Read the model definition and answer for the solid it produces. Units are mm, in the model's axes. A direction names the side the tool comes from. Coordinates: 2 decimals unless noted, no trailing zeros. Order: outer loops, then holes, each group sorted by start corner. A loop starts at its lowest first (then second) coordinate and runs counter-clockwise, first axis right, second up. Notation, with made-up numbers: (80, 12.5) -> (121, 12.5) arc R31 ccw to (121, 38.5) -> close; hole circle Ø6 at (72.25, 3.25). An arc over 180 degrees is marked (long way). Answer as a JSON object with one key per item and string values. Group by question number.
1) Determine the mould class of faces 3 (the flat face through (1.029, -5, 16)), 4 (the flat face through (-1, -1, 31.75)), 5 (the cylindrical face through (1.31, -7, 29.88)) for opening direction Z: released by +Z, released by -Z, zero draft, split by the parting line, or undercut.
2) Section C-C on y = -4.75 is taken. Determine the outline of the cut face in (x, z).
3) Consider L1, parallel to Z at x = 0, y = 1; L2, parallel to Y at x = -5.75, z = 17. Determine where each line is inside the solid, lowest interval first.
4) Given pin 1 (6.5 mm diameter, centred on x = -6, z = 16.5, fed in from -Y); pin 2 (2.5 mm diameter, centred on x = 0, y = -2, fed in from -Z); pin 3 (4 mm diameter, centred on y = -6, z = 13.5, fed in from -X), each flat-ended and moving along its own axis, determine where each tip first touches the part or whether it passes through.
5) Section D-D on z = 8.5 is taken. Determine the outline of the cut face in (x, y) (1 decimal).
6) Section A-A on z = 13.5 is taken. Determine the outline of the cut face in (x, y) (1 decimal).
7) A tool of negligible diameter and unlimited length cuts with its end or side. For faces 1 (the flat face through (-1, -1, 12.7)), 2 (the flat face through (1.588, -5, 16)), from which of +Z, -Z, +X, -X, +Y, -Y can it reach the whole face along a straight path? Write none if from no direction.
8) Section B-B on x = -2 is taken. Determine the outline of the cut face in (y, z), and give its area (3 significant figures).
from build123d import *

# Parameters (mm, degrees)
BOSS_EXTRUDE1_DEPTH = 31.75
SKETCH2_R           = 1.6383
SKETCH2_W           = 3.2131
SKETCH2_H           = 6.35
SKETCH2_W_2         = 1.5875
CUT_EXTRUDE1_DEPTH  = 4.826
SKETCH3_R           = 1.6383
CUT_EXTRUDE2_DEPTH  = 12.176
BOSS_EXTRUDE2_REACH = 21.05
SKETCH4_R           = 0.9525


with BuildPart() as part:
    # Sketch1 → Boss-Extrude1 (new body)
    with BuildSketch(Plane.XY):
        with BuildLine():
            Line((0, 1.5875), (-9.5885, 1.5875))
            Line((-9.5885, 1.5875), (-9.5885, 1.0287))
            Line((-9.5885, 1.0287), (-1.209104032, 1.0287))
            ThreePointArc((-1.209104032, 1.0287), (-1.122532015, -1.122532015), (1.0287, -1.209104032))
            Line((1.0287, -1.209104032), (1.0287, -9.5885))
            Line((1.0287, -9.5885), (1.5875, -9.5885))
            Line((1.5875, -9.5885), (1.5875, 0))
            ThreePointArc((1.5875, 0), (1.122532015, 1.122532015), (0, 1.5875))
        make_face()
    extrude(amount=BOSS_EXTRUDE1_DEPTH)

    # Sketch2 → Cut-Extrude1 (cut)
    with BuildSketch(Plane(origin=(0, 1.5875, 0), x_dir=(1, 0, 0), z_dir=(0, 1, 0))):
        with Locations((-6.0071, -28.575)):
            Circle(SKETCH2_R)
        with Locations((-6.0071, -3.175)):
            Circle(SKETCH2_R)
        with Locations((-1.60655, -15.875)):
            Rectangle(SKETCH2_W, SKETCH2_H)
        with Locations((0.79375, -15.875)):
            Rectangle(SKETCH2_W_2, SKETCH2_H)
    extrude(amount=-CUT_EXTRUDE1_DEPTH, mode=Mode.SUBTRACT)

    # Sketch3 → Cut-Extrude2 (cut, through all)
    with BuildSketch(Plane(origin=(1.5875, 0, 0), x_dir=(0, 0, -1), z_dir=(1, 0, 0))):
        with Locations((-28.575, -6.0071)):
            Circle(SKETCH3_R)
        with Locations((-3.175, -6.0071)):
            Circle(SKETCH3_R)
    extrude(amount=-CUT_EXTRUDE2_DEPTH, mode=Mode.SUBTRACT)

    # Sketch4 → Boss-Extrude2 (add, up to next)
    with BuildSketch(Plane(origin=(0, 0, 19.05), x_dir=(-1, 0, 0), z_dir=(0, 0, -1)), mode=Mode.PRIVATE) as boss_extrude2_sk1:
        Circle(SKETCH4_R)
    boss_extrude2_tool1 = extrude(boss_extrude2_sk1.sketch, amount=BOSS_EXTRUDE2_REACH, mode=Mode.PRIVATE) - part.part
    add(boss_extrude2_tool1.solids().sort_by_distance((0, 0, 19.05))[0])


solid = part.part
Worked answers:
{
 "1": {"face 3": "zero draft", "face 4": "released by +Z", "face 5": "undercut"},
 "2": {"outline": "(1.03, 0) -> (1.59, 0) -> (1.59, 2.12) -> (1.03, 2.12) -> close; (1.03, 4.23) -> (1.59, 4.23) -> (1.59, 27.52) -> (1.03, 27.52) -> close; (1.03, 29.63) -> (1.59, 29.63) -> (1.59, 31.75) -> (1.03, 31.75) -> close"},
 "3": {"L1": "z = 0 to 12.7, 19.05 to 31.75", "L2": "y = 1.03 to 1.59"},
 "4": {"pin 1": "stops at y = 1.03", "pin 2": "stops at z = 0", "pin 3": "stops at x = 1.03"},
 "5": {"outline": "(-9.6, 1) -> (-1.2, 1) arc R1.6 ccw to (1, -1.2) -> (1, -9.6) -> (1.6, -9.6) -> (1.6, 0) arc R1.6 ccw to (0, 1.6) -> (-9.6, 1.6) -> close"},
 "6": {"outline": "(-9.6, 1) -> (-3.2, 1) -> (-3.2, 1.6) -> (-9.6, 1.6) -> close; circle Ø1.9 at (0, 0); (1, -9.6) -> (1.6, -9.6) -> (1.6, -3.2) -> (1, -3.2) -> close"},
 "7": {"face 1": "none", "face 2": "+Z, -Z, +X, +Y, -Y"},
 "8": {"outline": "(1.03, 0) -> (1.59, 0) -> (1.59, 12.7) -> (1.03, 12.7) -> close; (1.03, 19.05) -> (1.59, 19.05) -> (1.59, 31.75) -> (1.03, 31.75) -> close", "area": "14.2 mm²"}
}
